Check sheet for the modelled part. Datum: model origin and axes. Units: mm. Face numbers are marked on the shaded views. Give positions to 0.01 mm unless a question says otherwise; leave off trailing zeros. Loops run counter-clockwise (first coordinate to the right, second up) from the corner with the lowest first, then second, coordinate; pieces in that order, holes last.
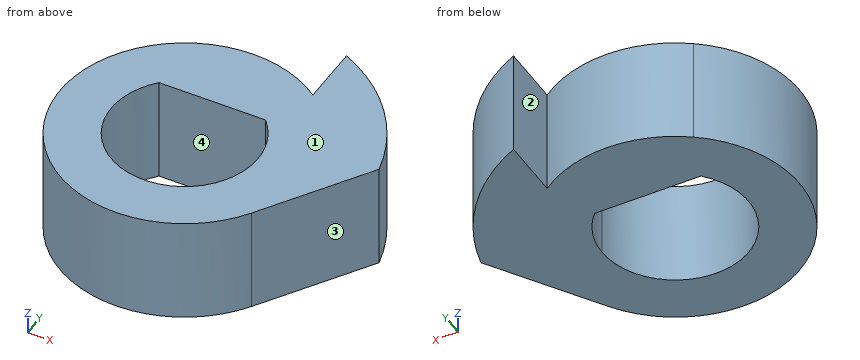
```python
from build123d import *

# Parameters (mm, degrees)
F1_DEPTH = 6


with BuildPart() as f1:
    # F0 (on Top) → F1 (new body)
    with BuildSketch(Plane.XY):
        with BuildLine():
            ThreePointArc((-4.125, 5.655473), (-4.812056, -5.083711), (5.873261, -3.808517))
            ThreePointArc((5.873261, -3.808517), (6.712408, -1.985846), (7, 0))
            ThreePointArc((7, 0), (6.239992, 3.172144), (4.125, 5.655473))
            ThreePointArc((4.125, 5.655473), (0, 7), (-4.125, 5.655473))
        make_face()
        with BuildLine():
            ThreePointArc((3, 2.831188), (3.833447, 1.523257), (4.125, 0))
            ThreePointArc((4.125, 0), (-1.523257, -3.833447), (-3, 2.831188))
            ThreePointArc((-3, 2.831188), (0, 4.125), (3, 2.831188))
        make_face(mode=Mode.SUBTRACT)
        with BuildLine():
            Line((-3, 2.831188), (3, 2.831188))
            ThreePointArc((3, 2.831188), (0, 4.125), (-3, 2.831188))
        make_face()
        with BuildLine():
            Line((5.873261, -3.808517), (9.758726, 2.183408))
            ThreePointArc((9.758726, 2.183408), (7.757732, 6.310118), (4.125, 9.109576))
            Line((4.125, 9.109576), (4.125, 5.655473))
            ThreePointArc((4.125, 5.655473), (6.239992, 3.172144), (7, 0))
            ThreePointArc((7, 0), (6.712408, -1.985846), (5.873261, -3.808517))
        make_face()
    extrude(amount=F1_DEPTH)


solid = f1.part
```
(1) Section check C-C on z = 2.2. Record the boundary of the cut face in (x, y) (3 decimals), plus the area to 3 significant figures.
(2) Section check D-D on y = 4.25. Record the boundary of the cut face in (x, z), plus the area to 3 significant figures.
(3) Section check B-B on x = 0. Record the boundary of the cut face in (y, z) (3 decimals).
(4) Gauge pin test, flat ends, axial feed: pin 1 Ø2 at (y, z) = (6.5, 4.5) entering from -X; pin 2 Ø1.5 at (x, z) = (-2, 5.5) entering from +Y. Record the tip position at first contact, or that the pin passes through.
(5) Release check for a two-part mould opening along X. For the marked faces 1, 2, 3 and 4 record: pulls with the +X half, pulls with the -X half, needs draft (parallel to the pull), parting line crosses it, or undercut.
(6) Material ranges on line 1 (Y direction, x = 0, z = 4.85) (3 decimals); line 2 (X direction, y = 8.25, z = 3.1) (3 decimals); line 3 (X direction, y = -0.25, z = 2), recorded low to high.
(7) Section check A-A on y = -0.75. Record the boundary of the cut face in (x, z), plus the area to 3 significant figures.
Computed values:
1. outline: (4.125, 5.655) arc R7 ccw (long way) to (5.873, -3.809) - (9.759, 2.183) arc R10 ccw to (4.125, 9.11) - close; hole (-3, 2.831) arc R4.125 ccw (long way) to (4.125, 0) arc R4.125 ccw to (3, 2.831) - close
1. area: 133 mm2
2. outline: (-5.56, 0) - (9.05, 0) - (9.05, 6) - (-5.56, 6) - close
2. area: 87.7 mm2
3. outline: (-7, 0) - (-4.125, 0) - (-4.125, 6) - (-7, 6) - close; (2.831, 0) - (7, 0) - (7, 6) - (2.831, 6) - close
4. pin 1: stops at x = -4.33
4. pin 2: stops at y = 6.89
5. face 1: needs draft
5. face 2: undercut
5. face 3: pulls with the +X half
5. face 4: undercut
6. line 1: y = -7 to -4.125, 2.831 to 7
6. line 2: x = 4.125 to 5.651
6. line 3: x = -7 to -4.12, 4.12 to 8.18
7. outline: (-6.96, 0) - (-4.06, 0) - (-4.06, 6) - (-6.96, 6) - close; (4.06, 0) - (7.86, 0) - (7.86, 6) - (4.06, 6) - close
7. area: 40.2 mm2
